The figure shows three views and two pictorial views of one solid part (mm, origin at its lowest corner). Answer the questions. A direction names the side the tool comes from. Give positions to 0.01 mm unless a question says otherwise; leave off trailing zeros. Order: outer loops, then holes, each group sorted by start corner. A loop starts at its lowest first (then second) coordinate and runs counter-clockwise, first axis right, second up. Notation, with made-up numbers: (21.25, 41.25) - (65.25, 41.25) arc R17 ccw to (65.25, 58.25) - close; hole circle Ø9 at (31.25, 81.5). An arc over 180 degrees is marked (long way). Use a Markdown table: item, result. Add a question column.
1. A cutting plane is placed at A-A on z = 30. Determine the outline of the cut face in (x, y).
2. Flat-ended cylindrical pins translate along their axes: P1, Ø12, axis at x = 45, z = 30, coming from the +Y side; P2, Ø11, axis at y = 47, z = 5, coming from the -X side; P3, Ø7.5, axis at x = 9.5, z = 29.5, coming from the +Y side; P4, Ø24, axis at x = 61.5, z = 22.5, coming from the -Y side. Find the tip coordinate at first contact, or state that the pin passes through.
3. For a pull along X with two mould halves and no side action, classify the marked faces 5, 6 and 7 as released by +X, released by -X, zero draft, split by the parting line, or undercut.
4. A cutting plane is placed at D-D on z = 12.5. Determine the outline of the cut face in (x, y), and give its area (4 significant figures).
5. A cutting plane is placed at B-B on y = 28. Determine the outline of the cut face in (x, z).
6. A cutting plane is placed at C-C on x = 29.5. Determine the outline of the cut face in (y, z), and give its area (3 significant figures).
7. Consider L1, parallel to X at y = 14.25, z = 30; L2, parallel to Z at x = 18.5, y = 2; L3, parallel to X at y = 32.5, z = 33.5. Determine where each line is inside the solid, lowest interval first.
8. Which of the six approach directions +Z, -Z, +X, -X, +Y, -Y give full straight-line access (tool end or side, diameter ignored) to the marked faces 1, 2, 3 and 4?
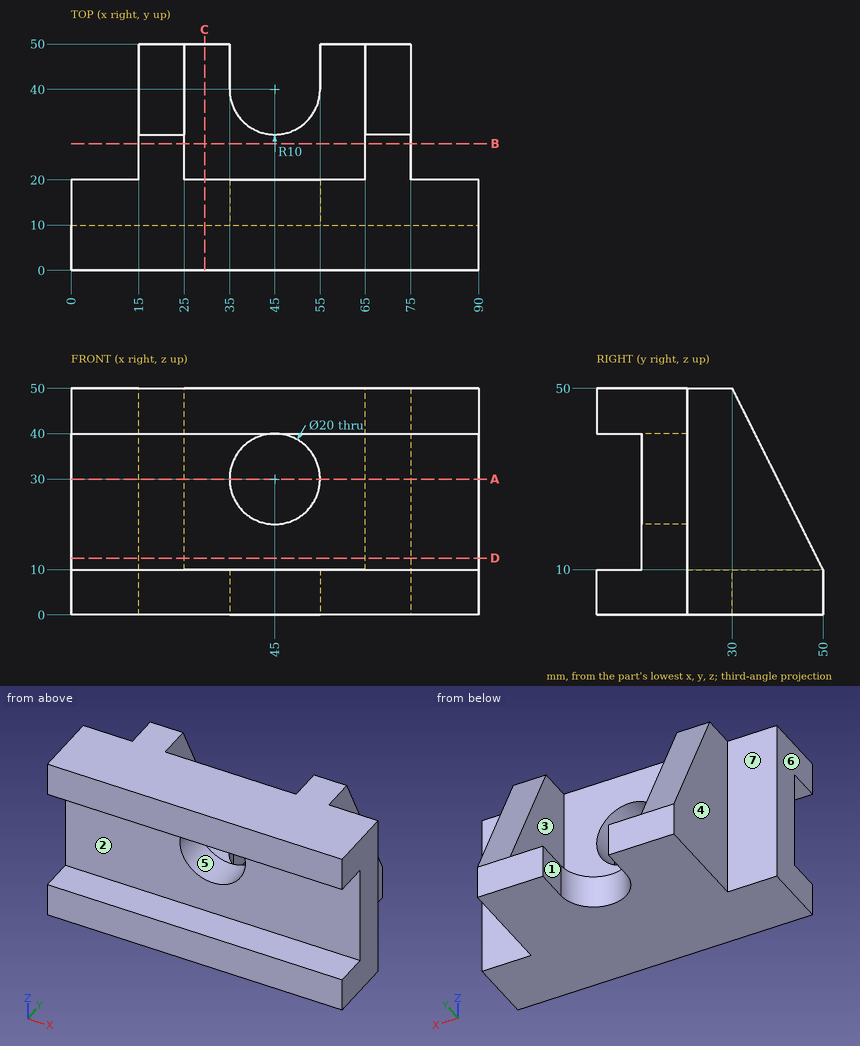
Output values:
| question | item | result |
|---|---|---|
| 1 | outline | (0, 10) - (35, 10) - (35, 20) - (25, 20) - (25, 40) - (15, 40) - (15, 20) - (0, 20) - close; (55, 10) - (90, 10) - (90, 20) - (75, 20) - (75, 40) - (65, 40) - (65, 20) - (55, 20) - close |
| 2 | P1 | through |
| 2 | P2 | x = 15 |
| 2 | P3 | y = 20 |
| 2 | P4 | y = 10 |
| 3 | face 5 | undercut |
| 3 | face 6 | released by -X |
| 3 | face 7 | zero draft |
| 4 | outline | (0, 10) - (90, 10) - (90, 20) - (75, 20) - (75, 48.75) - (65, 48.75) - (65, 20) - (25, 20) - (25, 48.75) - (15, 48.75) - (15, 20) - (0, 20) - close |
| 4 | area | 1,475 mm² |
| 5 | outline | (15, 0) - (75, 0) - (75, 50) - (65, 50) - (65, 10) - (25, 10) - (25, 50) - (15, 50) - close |
| 6 | outline | (0, 0) - (50, 0) - (50, 10) - (20, 10) - (20, 50) - (0, 50) - (0, 40) - (10, 40) - (10, 10) - (0, 10) - close |
| 6 | area | 1,000 mm² |
| 7 | L1 | 0 to 35, 55 to 90 |
| 7 | L2 | 0 to 10, 40 to 50 |
| 7 | L3 | 15 to 25, 65 to 75 |
| 8 | face 1 | +Z, -Z, +Y |
| 8 | face 2 | +X, -X, -Y |
| 8 | face 3 | +Z, +Y |
| 8 | face 4 | +Z, -Z, -X, +Y |
